Geometry check sheet. Reference: the model listing, model coordinates, mm. A direction names the side the tool comes from. Coordinates: 2 decimals unless noted, no trailing zeros. Order: outer loops, then holes, each group sorted by start corner. A loop starts at its lowest first (then second) coordinate and runs counter-clockwise, first axis right, second up.
```python
from build123d import *

# Parameters (mm, degrees)
SKETCH_1_R           = 5.5
EXTRUDE_1_DEPTH      = 6
EXTRUDE_2_DEPTH      = 4.5
EXTRUDE_2_DEPTH_BACK = 10.5
SKETCH_2_R           = 4.25
SKETCH_2_R_2         = 3
CUT_EXTRUDE_START    = -2
SKETCH_3_R           = 5.5
SKETCH_3_R_2         = 4.25
CUT_EXTRUDE_1_DEPTH  = 2


with BuildPart() as part:
    # 草图1 → 拉伸1 (new body)
    with BuildSketch(Plane(origin=(0, 0, 0), x_dir=(1, 0, 0), z_dir=(0, 1, 0))):
        with Locations(Location((0, 0, 0), (0, 0, 270))):
            Circle(SKETCH_1_R)
    extrude(amount=EXTRUDE_1_DEPTH)

    # 草图2 → 拉伸2 (add, two sides: drawn at the far end of the back side and taken through both)
    with BuildSketch(Plane(origin=(0, 6, 0), x_dir=(-1, 0, 0), z_dir=(0, 1, 0)).offset(-EXTRUDE_2_DEPTH_BACK)):
        with Locations(Location((0, 0, 0), (0, 0, 90))):
            Circle(SKETCH_2_R)
        with Locations(Location((0, 0, 0), (0, 0, 90))):
            Circle(SKETCH_2_R_2, mode=Mode.SUBTRACT)
    extrude(amount=EXTRUDE_2_DEPTH + EXTRUDE_2_DEPTH_BACK)

    # 草图3 → 切除-拉伸1 (cut)
    with BuildSketch(Plane(origin=(0, 4, 0), x_dir=(-1, 0, 0), z_dir=(0, 1, 0)).offset(CUT_EXTRUDE_START)):
        with Locations(Location((0, 0, 0), (0, 0, 90))):
            Circle(SKETCH_3_R)
        with Locations(Location((0, 0, 0), (0, 0, 90))):
            Circle(SKETCH_3_R_2, mode=Mode.SUBTRACT)
    extrude(amount=CUT_EXTRUDE_1_DEPTH, mode=Mode.SUBTRACT)


solid = part.part
```
Item 1: Tool access check on faces 1 (the face through (-5.37, 0.99, -1.19)), 2 (the face through (4.214, -2.282, -0.553)), 3 (the face through (-4, 2, 2)), 4 (the face through (-1, -4.5, -3)), 5 (the face through (0.9, 8.22, 2.86)). Record the directions out of +Z, -Z, +X, -X, +Y, -Y that give a thin tool (end or side, any length) a straight path to the whole face; none if there is none.
Item 2: Depth check by flat-ended pin: P1, Ø3, axis at x = -3, y = 8, coming from the +Z side; P2, Ø5.5, axis at x = 0, z = 0, coming from the -Y side; P3, Ø5, axis at x = -1, z = -1, coming from the +Y side; P4, Ø5, axis at x = 0, z = 0, coming from the +Y side. Enter the tip coordinate at first touch or a pass-through.
Item 3: Sectioned sample at C-C (y = 2.75). Record the cut outline in (x, z).
Item 4: Sectioned sample at A-A (z = 4.5). Record the cut outline in (x, y).
Item 5: Thickness scan on line 1 along Z through (x, y) = (0, 8.25); line 2 along Y through (x, z) = (5.25, 0). Record the ranges inside material, lowest first.
Item 6: Release check for a two-part mould opening along Z. For faces 6 (the face through (-5.37, 4.99, -1.19)), 7 (the face through (-1, 10.5, -3)), 8 (the face through (0, 6, 0)) record: pulls with the +Z half, pulls with the -Z half, needs draft (parallel to the pull), parting line crosses it, or undercut.
Item 7: Sectioned sample at B-B (x = 0). Record the cut outline in (y, z).
Item 8: Sectioned sample at D-D (z = 0). Record the cut outline in (x, y).
Geometry check:
1. face 1: +Y, -Y
1. face 2: -Y
1. face 3: none
1. face 4: +Z, -Z, +X, -X, -Y
1. face 5: +Y
2. P1: stops at z = 3.98
2. P2: stops at y = 0
2. P3: stops at y = 10.5
2. P4: stops at y = 6
3. outline: circle Ø8.5 at (0, 0)
4. outline: (-3.16, 0) - (3.16, 0) - (3.16, 2) - (-3.16, 2) - close; (-3.16, 4) - (3.16, 4) - (3.16, 6) - (-3.16, 6) - close
5. line 1: z = -4.25 to -3, 3 to 4.25
5. line 2: y = 0 to 2, 4 to 6
6. face 6: parting line crosses it
6. face 7: needs draft
6. face 8: undercut
7. outline: (-4.5, -4.25) - (0, -4.25) - (0, -5.5) - (2, -5.5) - (2, -4.25) - (4, -4.25) - (4, -5.5) - (6, -5.5) - (6, -4.25) - (10.5, -4.25) - (10.5, -3) - (6, -3) - (6, 3) - (10.5, 3) - (10.5, 4.25) - (6, 4.25) - (6, 5.5) - (4, 5.5) - (4, 4.25) - (2, 4.25) - (2, 5.5) - (0, 5.5) - (0, 4.25) - (-4.5, 4.25) - (-4.5, 3) - (0, 3) - (0, -3) - (-4.5, -3) - close
8. outline: (-5.5, 0) - (-4.25, 0) - (-4.25, -4.5) - (-3, -4.5) - (-3, 0) - (3, 0) - (3, -4.5) - (4.25, -4.5) - (4.25, 0) - (5.5, 0) - (5.5, 2) - (4.25, 2) - (4.25, 4) - (5.5, 4) - (5.5, 6) - (4.25, 6) - (4.25, 10.5) - (3, 10.5) - (3, 6) - (-3, 6) - (-3, 10.5) - (-4.25, 10.5) - (-4.25, 6) - (-5.5, 6) - (-5.5, 4) - (-4.25, 4) - (-4.25, 2) - (-5.5, 2) - close
